Read the model definition and answer for the solid it produces. Units are mm, in the model's axes. Face numbers are marked on the shaded views. A direction names the side the tool comes from. Give positions to 0.01 mm unless a question says otherwise; leave off trailing zeros. Loops run counter-clockwise (first coordinate to the right, second up) from the corner with the lowest first, then second, coordinate; pieces in that order, holes last. Notation, with made-up numbers: (-34, 43) - (19, 43) arc R22 ccw to (19, 69) - close; hole circle Ø6 at (-26, 38). An arc over 180 degrees is marked (long way). Write item = value, one per line.
```python
from build123d import *

# Parameters (mm, degrees)
F0_R            = 1
F1_DEPTH        = 6.5
F2_R            = 3.5
F3_DEPTH        = 4
F5_DEPTH        = 10.501
F5_COPIES_COUNT = 30


# Not quite as in the source:
# - a pattern or mirror of a feature is missing from the dataset's text; its kind, count and spacing are read off the source's solid


with BuildPart() as f1:
    # F0 (on Front) → F1 (new body)
    with BuildSketch(Plane.XZ):
        Circle(F0_R)
    extrude(amount=F1_DEPTH)

    # F2 (on face) → F3 (join)
    with BuildSketch(Plane(origin=(0, 0, 0), x_dir=(-1, 0, 0), z_dir=(0, 1, 0))):
        Circle(F2_R)
    extrude(amount=F3_DEPTH)

    # F4 (on face) → F5 (cut, through all)
    with BuildSketch(Plane(origin=(0, 4, 0), x_dir=(-1, 0, 0), z_dir=(0, 1, 0))):
        with BuildLine():
            Line((3.2, 0), (3.4881207588, -0.2881207588))
            ThreePointArc((3.4881207588, -0.2881207588), (3.5, 0), (3.4881207588, 0.2881207588))
            Line((3.4881207588, 0.2881207588), (3.2, 0))
        make_face()
    f5 = extrude(amount=-F5_DEPTH, mode=Mode.SUBTRACT)

    # F5_copies: F5 ×30 about axis
    f5_copies_axis = Axis((0, 0, 0), (0, 1, 0))
    for i in range(1, F5_COPIES_COUNT):
        add(f5.rotate(f5_copies_axis, i * 360 / F5_COPIES_COUNT), mode=Mode.SUBTRACT)


solid = f1.part
```
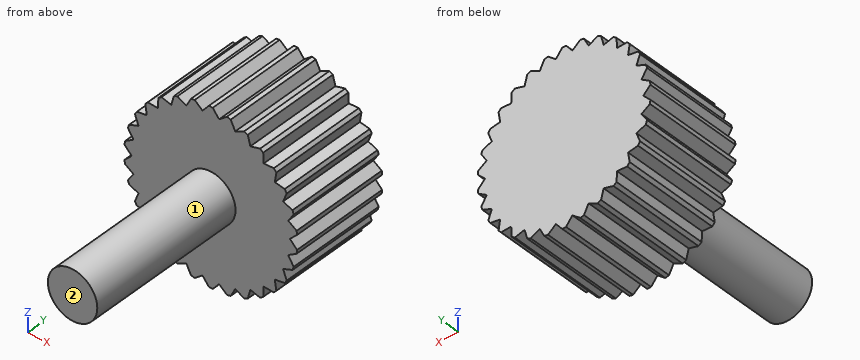
1) Each of these flat-tipped pins is pushed along its axis until it touches: P1, Ø2, axis at y = -4, z = 0, coming from the -X side; P2, Ø2, axis at y = -4, z = -1.5, coming from the -X side; P3, Ø1.5, axis at x = -2, z = 2, coming from the -Y side. Where does it stop, or does it pass through?
Output:
P1 = -1
P2 = -0.87
P3 = 0
2) A cutting plane is placed at C-C on z = 1.5. Determine the outline of the cut face in (x, y).
Output:
outline = (-3, 0) - (3, 0) - (3, 4) - (-3, 4) - close
3) A cutting plane is placed at B-B on y = -2.5. Determine the outline of the cut face in (x, z).
Output:
outline = circle Ø2 at (0, 0)
4) A tool of negligible diameter and unlimited length cuts with its end or side. For the marked faces 1 and 2, from which of +Z, -Z, +X, -X, +Y, -Y can it reach the whole face along a straight path? Write none if from no direction.
Output:
face_1 = -Y
face_2 = +Z, -Z, +X, -X, -Y
5) A cutting plane is placed at A-A on x = -0.5. Determine the outline of the cut face in (y, z).
Output:
outline = (-6.5, -0.87) - (0, -0.87) - (0, -3.32) - (4, -3.32) - (4, 3.32) - (0, 3.32) - (0, 0.87) - (-6.5, 0.87) - close
6) Find the intervals of material crossed by probe 1 along Y at (x, z) = (1.25, -0.5); probe 2 along Z at (x, y) = (-0.75, 1.5); probe 3 along X at (y, z) = (3.25, -0.25), in increasing order.
Output:
probe_1 = 0 to 4
probe_2 = -3.42 to 3.42
probe_3 = -3.45 to 3.45
